```python
from build123d import *

# Parameters (mm, degrees)
SKETCH013_R     = 3.5
SKETCH013_R_2   = 1.6
SKETCH013_W     = 7
SKETCH013_H     = 7
PAD004_DEPTH    = 3.5
PAD_DEPTH       = 10
SKETCH015_R     = 0.75
POCKET005_DEPTH = 7.5
SKETCH004_R     = 0.75
POCKET006_DEPTH = 10
SKETCH014_R     = 1.75
POCKET007_DEPTH = 5
POCKET_DEPTH    = 2


with BuildPart() as part:
    # Sketch013 → Pad004 (new body)
    with BuildSketch(Plane.XY):
        Polygon((0, 70), (150, 70.000096), (150, -70), (0, -70), align=None)
        with Locations((13, 25)):
            Circle(SKETCH013_R, mode=Mode.SUBTRACT)
        with Locations((58, 25)):
            Circle(SKETCH013_R, mode=Mode.SUBTRACT)
        with Locations((13, -30)):
            Circle(SKETCH013_R, mode=Mode.SUBTRACT)
        with Locations((58, -30)):
            Circle(SKETCH013_R, mode=Mode.SUBTRACT)
        with Locations((146, 66.000096)):
            Circle(SKETCH013_R_2, mode=Mode.SUBTRACT)
        with Locations((146, -66)):
            Circle(SKETCH013_R_2, mode=Mode.SUBTRACT)
        with Locations((81.000022, 43.53967)):
            Circle(SKETCH013_R_2, mode=Mode.SUBTRACT)
        with Locations((136, 43.53967)):
            Circle(SKETCH013_R_2, mode=Mode.SUBTRACT)
        with Locations((80.901087, -46.460276)):
            Circle(SKETCH013_R_2, mode=Mode.SUBTRACT)
        with Locations((135.901066, -46.460276)):
            Circle(SKETCH013_R_2, mode=Mode.SUBTRACT)
        with Locations((90.500022, 43.53967)):
            Rectangle(SKETCH013_W, SKETCH013_H, mode=Mode.SUBTRACT)
        with Locations((108.500011, 43.519883)):
            Rectangle(SKETCH013_W, SKETCH013_H, mode=Mode.SUBTRACT)
        with Locations((126.5, 43.500096)):
            Rectangle(SKETCH013_W, SKETCH013_H, mode=Mode.SUBTRACT)
        with Locations((90.480235, 25.539681)):
            Rectangle(SKETCH013_W, SKETCH013_H, mode=Mode.SUBTRACT)
        with Locations((108.480224, 25.519894)):
            Rectangle(SKETCH013_W, SKETCH013_H, mode=Mode.SUBTRACT)
        with Locations((126.480213, 25.500107)):
            Rectangle(SKETCH013_W, SKETCH013_H, mode=Mode.SUBTRACT)
        with Locations((90.460448, 7.539692)):
            Rectangle(SKETCH013_W, SKETCH013_H, mode=Mode.SUBTRACT)
        with Locations((108.460437, 7.519905)):
            Rectangle(SKETCH013_W, SKETCH013_H, mode=Mode.SUBTRACT)
        with Locations((126.460426, 7.500118)):
            Rectangle(SKETCH013_W, SKETCH013_H, mode=Mode.SUBTRACT)
        with Locations((90.440661, -10.460297)):
            Rectangle(SKETCH013_W, SKETCH013_H, mode=Mode.SUBTRACT)
        with Locations((108.44065, -10.480084)):
            Rectangle(SKETCH013_W, SKETCH013_H, mode=Mode.SUBTRACT)
        with Locations((126.440639, -10.499871)):
            Rectangle(SKETCH013_W, SKETCH013_H, mode=Mode.SUBTRACT)
        with Locations((90.420874, -28.460286)):
            Rectangle(SKETCH013_W, SKETCH013_H, mode=Mode.SUBTRACT)
        with Locations((108.420863, -28.480073)):
            Rectangle(SKETCH013_W, SKETCH013_H, mode=Mode.SUBTRACT)
        with Locations((126.420852, -28.49986)):
            Rectangle(SKETCH013_W, SKETCH013_H, mode=Mode.SUBTRACT)
        with Locations((90.401087, -46.460276)):
            Rectangle(SKETCH013_W, SKETCH013_H, mode=Mode.SUBTRACT)
        with Locations((108.401076, -46.480062)):
            Rectangle(SKETCH013_W, SKETCH013_H, mode=Mode.SUBTRACT)
        with Locations((126.401066, -46.499849)):
            Rectangle(SKETCH013_W, SKETCH013_H, mode=Mode.SUBTRACT)
    extrude(amount=PAD004_DEPTH)

    # Sketch001 → Pad (join)
    with BuildSketch(Plane.XY.offset(3.5)):
        Polygon((0, 60), (3, 60), (128, 60), (128, 57), (3, 57), (3, -67), (128, -67), (128, -70), (3, -70), (0, -70), align=None)
    extrude(amount=PAD_DEPTH)

    # Sketch015 → Pocket005 (cut, symmetric)
    with BuildSketch(Plane.XZ.offset(65)):
        with Locations((53, 7)):
            Circle(SKETCH015_R)
    extrude(amount=POCKET005_DEPTH, both=True, mode=Mode.SUBTRACT)

    # Sketch004 → Pocket006 (cut, symmetric)
    with BuildSketch(Plane.XZ.offset(-55)):
        with Locations((25, 9)):
            Circle(SKETCH004_R)
        with Locations((95, 9)):
            Circle(SKETCH004_R)
        with Locations((55, 9)):
            Circle(SKETCH004_R)
        with Locations((125, 9)):
            Circle(SKETCH004_R)
    extrude(amount=POCKET006_DEPTH, both=True, mode=Mode.SUBTRACT)

    # Sketch014 → Pocket007 (cut)
    with BuildSketch(Plane.YZ):
        with Locations((45, 8)):
            Circle(SKETCH014_R)
        with Locations((-5, 8)):
            Circle(SKETCH014_R)
        with Locations((-55, 8)):
            Circle(SKETCH014_R)
    extrude(amount=POCKET007_DEPTH, mode=Mode.SUBTRACT)

    # Sketch → Pocket (cut)
    with BuildSketch(Plane.XY.offset(3.5)):
        Polygon((83.55, 52), (134.15, 52), (134.15, 40), (140, 40), (140, -42.5), (134.15, -42.5), (134.15, -53), (83.55, -53), (83.55, -42.5), (72.55, -42.5), (72.55, 40), (83.55, 40), align=None)
    extrude(amount=-POCKET_DEPTH, mode=Mode.SUBTRACT)


solid = part.part
```
The listing builds one solid part. Answer for the finished solid, in the listing's coordinates (mm). A direction names the side the tool comes from. Give positions to 0.01 mm unless a question says otherwise; leave off trailing zeros. Order: outer loops, then holes, each group sorted by start corner. A loop starts at its lowest first (then second) coordinate and runs counter-clockwise, first axis right, second up. Notation, with made-up numbers: (-39.75, 33) - (4.25, 33) arc R27 ccw to (4.25, 64) - close; hole circle Ø2 at (86.5, -19.75). An arc over 180 degrees is marked (long way). Use one line per item in the form item = value. Start each with the question number.
(1) Flat-ended cylindrical pins translate along their axes: pin 1 Ø4 at (x, z) = (37, 11) entering from +Y; pin 2 Ø1.5 at (y, z) = (-69, 7.5) entering from +X; pin 3 Ø8 at (x, y) = (75.5, -48.5) entering from +Z. Find the tip coordinate at first contact, or state that the pin passes through.
(2) The mould has two halves that part along Y. Classify faces 1 (the cylindrical face through (134.63, -47.43, 1.73)), 2 (the flat face through (2.7, -4.7, 13.5)), 3 (the flat face through (74, -70, 7)): released by +Y, released by -Y, zero draft, split by the parting line, or undercut.
(3) Consider line 1 (Y direction, x = 146, z = 1.2); line 2 (Y direction, x = 75.5, z = 7.75); line 3 (X direction, y = -25.5, z = 2.5). Determine where each line is inside the solid, lowest interval first. Write a range as from..to.
(4) For faces 4 (the flat face through (0, -1, 7)), 5 (the flat face through (65, 60, 8)), 6 (the flat face through (3, -4, 10)), determine the directions among +Z, -Z, +X, -X, +Y, -Y from which every point of the face is accessible in a straight line to the end or side of a thin tool.
(5) A cutting plane is placed at D-D, the plane y = 33.5. Write down the section's boundary in (x, z).
(6) A cutting plane is placed at B-B, the plane z = 11.5. Write down the section's boundary in (x, y).
(7) A cutting plane is placed at A-A, the plane y = -5. Write down the section's boundary in (x, z), then the cut area to 3 significant figures.
(8) A cutting plane is placed at C-C, the plane x = 40. Write down the section's boundary in (y, z).
Ans:
q1.pin_1 = 60
q1.pin_2 = 128
q1.pin_3 = 3.5
q2.face_1 = undercut
q2.face_2 = zero draft
q2.face_3 = released by -Y
q3.line_1 = -70..-67.6, -64.4..64.4, 67.6..70
q3.line_2 = -70..-67, 57..60
q3.line_3 = 0..72.55, 140..150
q4.face_4 = +Z, -Z, -X, +Y, -Y
q4.face_5 = +Z, +X, -X, +Y
q4.face_6 = +Z, +X
q5.outline = (0, 0) - (150, 0) - (150, 3.5) - (140, 3.5) - (140, 1.5) - (72.55, 1.5) - (72.55, 3.5) - (3, 3.5) - (3, 13.5) - (0, 13.5) - close
q6.outline = (0, -70) - (128, -70) - (128, -67) - (3, -67) - (3, 57) - (128, 57) - (128, 60) - (0, 60) - close
q7.outline = (0, 0) - (150, 0) - (150, 3.5) - (140, 3.5) - (140, 1.5) - (72.55, 1.5) - (72.55, 3.5) - (3, 3.5) - (3, 6.25) - (0, 6.25) - close; (0, 9.75) - (3, 9.75) - (3, 13.5) - (0, 13.5) - close
q7.area = 410 mm^2
q8.outline = (-70, 0) - (70, 0) - (70, 3.5) - (60, 3.5) - (60, 13.5) - (57, 13.5) - (57, 3.5) - (-67, 3.5) - (-67, 13.5) - (-70, 13.5) - close
